Input: part model. Units: mm. Frame: model coordinates. Face numbers are marked on the shaded views. A direction names the side the tool comes from. Coordinates: 2 decimals unless noted, no trailing zeros. Loops run counter-clockwise (first coordinate to the right, second up) from the corner with the lowest first, then second, coordinate; pieces in that order, holes last. Notation, with made-up numbers: (70.5, -12.75) - (86.5, -12.75) arc R25 ccw to (86.5, 8.25) - close; hole circle Ø8 at (0, 80). An arc over 180 degrees is marked (long way). Answer as CSV lines item,"result". Start each with the question number.
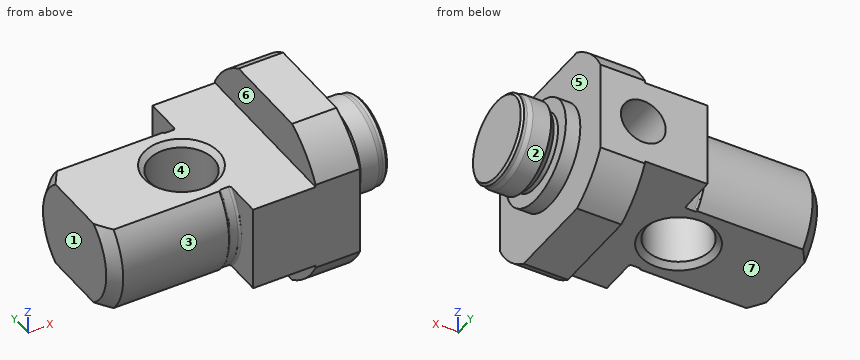
```python
from build123d import *

# Parameters (mm, degrees)
O_L_DEPTH             = 17.85
CUT_EXTRUDE4_REACH    = 17
CUT_EXTRUDE2_REACH    = 13.95
SKETCH4_R             = 3
CHAMFER4_SIZE         = 0.5
M5_TAPPED_HOLE1_D     = 4.2
M5_TAPPED_HOLE1_DEPTH = 6
M5_TAPPED_HOLE1_TIP   = 1.212435565


with BuildPart() as part:
    # Sketch1 → Revolve1 (revolve)
    with BuildSketch(Plane.XY):
        with BuildLine():
            Line((-22, 0), (-22, 5))
            Line((-22, 5), (-21, 6))
            Line((-21, 6), (-11.1, 6))
            Line((-11.1, 6), (-11.058578644, 5.958578644))
            ThreePointArc((-11.058578644, 5.958578644), (-10.993693974, 5.915224093), (-10.917157288, 5.9))
            Line((-10.917157288, 5.9), (-10.2, 5.9))
            ThreePointArc((-10.2, 5.9), (-10.058578644, 5.958578644), (-10, 6.1))
            Line((-10, 6.1), (-10, 9))
            Line((-10, 9), (0, 9))
            Line((0, 9), (0, 4.75))
            Line((0, 4.75), (1.35, 4.75))
            Line((1.35, 4.75), (1.35, 3.5))
            Line((1.35, 3.5), (1.75, 3.5))
            Line((1.75, 3.5), (2.35, 4.1))
            Line((2.35, 4.1), (4.052153903, 4.1))
            Line((4.052153903, 4.1), (4.5, 3.98))
            Line((4.5, 3.98), (4.8, 3.98))
            Line((4.8, 3.98), (5, 3.78))
            Line((5, 3.78), (5, 0))
            Line((5, 0), (-22, 0))
        make_face()
    revolve(axis=Axis((0, 0, 0), (1, 0, 0)))

    # Sketch3 → O-L (cut)
    with BuildSketch(Plane.ZY.offset(22)):
        with BuildLine():
            Line((-4, 8.062257748), (-4, -8.062257748))
            ThreePointArc((-4, -8.062257748), (-9, 0), (-4, 8.062257748))
        make_face()
        with BuildLine():
            Line((4, 8.062257748), (4, -8.062257748))
            ThreePointArc((4, -8.062257748), (9, 0), (4, 8.062257748))
        make_face()
    extrude(amount=-O_L_DEPTH, mode=Mode.SUBTRACT)

    # Sketch6 → Cut-Extrude4 (cut, up to next)
    with BuildSketch(Plane.ZY.offset(10), mode=Mode.PRIVATE) as cut_extrude4_sk1:
        with BuildLine():
            Line((-4.218708333, 7.95), (4.218708333, 7.95))
            ThreePointArc((4.218708333, 7.95), (0, 9), (-4.218708333, 7.95))
        make_face()
    cut_extrude4_tool1 = extrude(cut_extrude4_sk1.sketch, amount=-CUT_EXTRUDE4_REACH, mode=Mode.PRIVATE) & part.part
    add(cut_extrude4_tool1.solids().sort_by_distance((-10, 8.372173, 0))[0], mode=Mode.SUBTRACT)
    # Sketch6 → Cut-Extrude4 (cut, up to next)
    with BuildSketch(Plane.ZY.offset(10), mode=Mode.PRIVATE) as cut_extrude4_sk2:
        with BuildLine():
            Line((7.95, 4.218708333), (7.95, -4.218708333))
            ThreePointArc((7.95, -4.218708333), (9, 0), (7.95, 4.218708333))
        make_face()
    cut_extrude4_tool2 = extrude(cut_extrude4_sk2.sketch, amount=-CUT_EXTRUDE4_REACH, mode=Mode.PRIVATE) & part.part
    add(cut_extrude4_tool2.solids().sort_by_distance((-10, 0, 8.372173))[0], mode=Mode.SUBTRACT)
    # Sketch6 → Cut-Extrude4 (cut, up to next)
    with BuildSketch(Plane.ZY.offset(10), mode=Mode.PRIVATE) as cut_extrude4_sk3:
        with BuildLine():
            Line((4.218708333, -7.95), (-4.218708333, -7.95))
            ThreePointArc((-4.218708333, -7.95), (0, -9), (4.218708333, -7.95))
        make_face()
    cut_extrude4_tool3 = extrude(cut_extrude4_sk3.sketch, amount=-CUT_EXTRUDE4_REACH, mode=Mode.PRIVATE) & part.part
    add(cut_extrude4_tool3.solids().sort_by_distance((-10, -8.372173, 0))[0], mode=Mode.SUBTRACT)
    # Sketch6 → Cut-Extrude4 (cut, up to next)
    with BuildSketch(Plane.ZY.offset(10), mode=Mode.PRIVATE) as cut_extrude4_sk4:
        with BuildLine():
            Line((-7.95, -4.218708333), (-7.95, 4.218708333))
            ThreePointArc((-7.95, 4.218708333), (-9, 0), (-7.95, -4.218708333))
        make_face()
    cut_extrude4_tool4 = extrude(cut_extrude4_sk4.sketch, amount=-CUT_EXTRUDE4_REACH, mode=Mode.PRIVATE) & part.part
    add(cut_extrude4_tool4.solids().sort_by_distance((-10, 0, -8.372173))[0], mode=Mode.SUBTRACT)

    # Sketch4 → Cut-Extrude2 (cut, up to next)
    with BuildSketch(Plane.XY.offset(4), mode=Mode.PRIVATE) as cut_extrude2_sk1:
        with Locations((-12, 0)):
            Circle(SKETCH4_R)
    cut_extrude2_tool1 = extrude(cut_extrude2_sk1.sketch, amount=-CUT_EXTRUDE2_REACH, mode=Mode.PRIVATE) & part.part
    add(cut_extrude2_tool1.solids().sort_by_distance((-12, 0, 4))[0], mode=Mode.SUBTRACT)

    # Chamfer4
    chamfer4_edges = [part.edges().sort_by_distance(p)[0] for p in [
        (-15, 0, 4),
        (-15, 0, -4),
    ]]
    chamfer(chamfer4_edges, length=CHAMFER4_SIZE)

    # M5 Tapped Hole1
    with Locations(Plane(origin=(0, 7.95, 0), x_dir=(1, 0, 0), z_dir=(0, 1, 0))):
        with Locations((-4, 0)):
            Hole(M5_TAPPED_HOLE1_D / 2, depth=M5_TAPPED_HOLE1_DEPTH)
            with Locations((0, 0, -(M5_TAPPED_HOLE1_DEPTH + M5_TAPPED_HOLE1_TIP / 2))):  # 120° drill point
                Cone(0, M5_TAPPED_HOLE1_D / 2, M5_TAPPED_HOLE1_TIP, mode=Mode.SUBTRACT)


solid = part.part
```
Item 1: Draft query along Y for the marked faces 1, 2, 3 and 4. Return one class per face: pulls with the +Y half, pulls with the -Y half, needs draft (parallel to the pull), parting line crosses it, or undercut.
Item 2: Section query C-C, the plane y = 1.5. Give the number of separate pieces and of enclosed holes in the cut face, and give its area (3 significant figures).
Item 3: Material intervals for probe 1 along X at (y, z) = (-3.25, 1.75); probe 2 along Z at (x, y) = (-4, 3.75); probe 3 along Z at (x, y) = (-16.5, 4.25), sorted ascending.
Item 4: Section query A-A, the plane x = -12. Output: boundary loops of the cut face in (y, z).
Item 5: Set-up query: the marked faces 5, 6 and 7. Return all of +Z, -Z, +X, -X, +Y, -Y with unobstructed straight access to the full face (end or side cutting, diameter ignored); none if empty.
Item 6: Section query B-B, the plane y = -7. Output: boundary loops of the cut face in (x, z).
Item 7: Section query D-D, the plane x = 3. Output: boundary loops of the cut face in (y, z).
Item 8: Contact query for flat-ended pins moving along their axis: P1, Ø8, axis at x = -9.5, y = 1, coming from the +Z side; P2, Ø4.5, axis at y = -2.5, z = -6.5, coming from the -X side; P3, Ø4, axis at x = -7, y = 3, coming from the -Z side. Output: stop coordinate, or through.
Response values:
1,face 1,"needs draft"
1,face 2,"parting line crosses it"
1,face 3,"pulls with the -Y half"
1,face 4,"undercut"
2,separate pieces,"2"
2,enclosed holes,"1"
2,area,"200 mm²"
3,probe 1,"x = -22 to 1.35, 1.94 to 5"
3,probe 2,"z = -7.95 to -2.1, 2.1 to 7.95"
3,probe 3,"z = -4 to 4"
4,outline,"(-4.47, -4) - (-3.5, -4) - (-3, -3.5) - (-3, 3.5) - (-3.5, 4) - (-4.47, 4) arc R6 ccw to start; (3, -3.5) - (3.5, -4) - (4.47, -4) arc R6 ccw to (4.47, 4) - (3.5, 4) - (3, 3.5) - close"
5,face 5,"+X"
5,face 6,"+Z, -X, +Y, -Y"
5,face 7,"-Z, -X, +Y, -Y"
6,outline,"(-10, -4) - (-4.15, -4) - (-4.15, -5.66) - (0, -5.66) - (0, 5.66) - (-4.15, 5.66) - (-4.15, 4) - (-10, 4) - close"
7,outline,"circle Ø8.2 at (0, 0)"
8,P1,"stops at z = 4"
8,P2,"stops at x = -4.15"
8,P3,"stops at z = -4"
